Part model, mm, in its own coordinate system. A direction names the side the tool comes from. Round coordinates to 2 decimals unless told otherwise and drop trailing zeros. Use one line per item in the form item = value. Start each with the question number.
Item 1: Which spindle directions (+Z, -Z, +X, -X, +Y, -Y) get a long thin tool onto all of the face, cutting with end or side? Do faces 4 (the face through (237, -25, 25)), 5 (the face through (14.807, -25.35, 20.564)). Say none if no direction does.
Item 2: Probe L1, parallel to X at y = -35.5, z = -25.5; L2, parallel to Z at x = 12.5, y = -32; L3, parallel to X at y = -23, z = 26. List the from-to ranges inside material, lowest first.
Item 3: Mould opens along X. For faces 1 (the face through (287, -25, 25)), 2 (the face through (-4, -25, -50)), 3 (the face through (312.5, -25, -1)) say: +X half, -X half, draft (parallel to the pull), parting line (faces both ways), or undercut.
from build123d import *

# Parameters (mm, degrees)
F0_W     = 625
F0_H     = 100
F1_DEPTH = 50
F2_R     = 5
F3_DEPTH = 50
F4_R     = 5
F5_DEPTH = 25


with BuildPart() as f1:
    # F0 (on Front) → F1 (new body)
    with BuildSketch(Plane.XZ):
        Rectangle(F0_W, F0_H)
    extrude(amount=F1_DEPTH)

    # F2 (on face) → F3 (cut)
    with BuildSketch(Plane.XZ.offset(50)):
        with Locations((-37.5, -25)):
            Circle(F2_R)
        with Locations((12.5, -25)):
            Circle(F2_R)
        with Locations((-37.5, 25)):
            Circle(F2_R)
        with Locations((12.5, 25)):
            Circle(F2_R)
    extrude(amount=-F3_DEPTH, mode=Mode.SUBTRACT)

    # F4 (on face) → F5 (cut)
    with BuildSketch(Plane.XY.offset(50)):
        with Locations((237.5, -25)):
            Circle(F4_R)
        with Locations((287.5, -25)):
            Circle(F4_R)
    extrude(amount=-F5_DEPTH, mode=Mode.SUBTRACT)


solid = f1.part
Model answer:
q1.face_4 = +Z
q1.face_5 = +Y, -Y
q2.L1 = -312.5 to -42.47, -32.53 to 7.53, 17.47 to 312.5
q2.L2 = -50 to -30, -20 to 20, 30 to 50
q2.L3 = -312.5 to -42.4, -32.6 to 7.6, 17.4 to 232.92, 242.08 to 282.92, 292.08 to 312.5
q3.face_1 = undercut
q3.face_2 = draft
q3.face_3 = +X half
